Build history of the part. All positions in model axes, mm. A direction names the side the tool comes from. Coordinates: 2 decimals unless noted, no trailing zeros. Order: outer loops, then holes, each group sorted by start corner. A loop starts at its lowest first (then second) coordinate and runs counter-clockwise, first axis right, second up. Notation, with made-up numbers: (-7, -31) - (6, -31) arc R16 cw to (6, -18) - close; hole circle Ø6 at (58.25, -11.5). An arc over 180 degrees is marked (long way). Return JSON: item names as keys, results as strings.
from build123d import *

# Parameters (mm, degrees)
SKETCH1_W           = 3
SKETCH1_H           = 2.75
SKETCH2_R           = 1.5
BOSS_EXTRUDE1_DEPTH = 30
CUT_EXTRUDE1_DEPTH  = 1.5
CHAMFER1_SIZE       = 0.3


with BuildPart() as part:
    # Sketch1 → Revolve1 (revolve)
    with BuildSketch(Plane.XY, mode=Mode.PRIVATE) as revolve1_sk:
        with Locations((-1.5, 1.375)):
            Rectangle(SKETCH1_W, SKETCH1_H)
    revolve(revolve1_sk.sketch.rotate(Axis((-3, 0, 0), (1, 0, 0)), 270), axis=Axis((-3, 0, 0), (1, 0, 0)))

    # Sketch2 → Boss-Extrude1 (add)
    with BuildSketch(Plane(origin=(0, 0, 0), x_dir=(0, 0, -1), z_dir=(1, 0, 0))):
        Circle(SKETCH2_R)
    extrude(amount=BOSS_EXTRUDE1_DEPTH)

    # Sketch3 → Cut-Extrude1 (cut)
    with BuildSketch(Plane.ZY.offset(3)):
        Polygon((1.25, -0.721687836), (1.25, 0.721687836), (0, 1.443375673), (-1.25, 0.721687836), (-1.25, -0.721687836), (0, -1.443375673), align=None)
    extrude(amount=-CUT_EXTRUDE1_DEPTH, mode=Mode.SUBTRACT)

    # Sketch4 → Cut-Revolve1 (revolve, cut)
    with BuildSketch(Plane.XY, mode=Mode.PRIVATE) as cut_revolve1_sk:
        Polygon((-1.5, 1.25), (-1.5, 0), (-1.165063509, 0), align=None)
    revolve(cut_revolve1_sk.sketch.rotate(Axis((-1.500025, 0, 0), (1, 0, 0)), 90), axis=Axis((-1.500025, 0, 0), (1, 0, 0)), mode=Mode.SUBTRACT)

    # Chamfer1
    chamfer1_edges = [part.edges().sort_by_distance(p)[0] for p in [
        (-3, 0, 2.75),
        (30, 0, 1.5),
    ]]
    chamfer(chamfer1_edges, length=CHAMFER1_SIZE)


solid = part.part
1. Tool access for faces 1 (the flat face through (-2, 0, 1.25)), 2 (the flat face through (30, 0, 0)), 3 (the flat face through (0, -1.2, 1.2)): list every direction of +Z, -Z, +X, -X, +Y, -Y with a clear straight run to the whole face (end or side of a thin tool).
Check values:
{"face 1": "-X", "face 2": "+Z, -Z, +X, +Y, -Y", "face 3": "+X"}
2. Mould opens along Z. For faces 4 (the flat face through (-3, -1.1, 1.1)), 5 (the flat face through (-2, 0, -1.25)), 6 (the cylindrical face through (-1.331, -2.685, 0.596)) say: pulls with the +Z half, pulls with the -Z half, needs draft (parallel to the pull), parting line crosses it, or undercut.
Check values:
{"face 4": "needs draft", "face 5": "undercut", "face 6": "parting line crosses it"}
3. Cut at A-A on x = 28. Give the cut face in (y, z).
Check values:
{"outline": "circle Ø3 at (0, 0)"}
4. Probe L1, parallel to X at y = 2, z = 1.1; L2, parallel to Y at x = 5, z = -0.9. List the from-to ranges inside material, lowest first.
Check values:
{"L1": "-3 to 0", "L2": "-1.2 to 1.2"}
5. Drop flat-ended pins along their axis: pin 1 (1.5 mm diameter, centred on x = 8.5, y = -1.5, fed in from -Z); pin 2 (1 mm diameter, centred on x = 15, y = -1.5, fed in from +Z); pin 3 (0.7 mm diameter, centred on x = -2.5, y = 0.5, fed in from +Z). Give the stop position or say it passes through.
Check values:
{"pin 1": "z = -1.3", "pin 2": "z = 1.12", "pin 3": "z = 2.75"}
